```python
from build123d import *

# Parameters (mm, degrees)
F1_DEPTH       = 13
F4_DEPTH       = 3
F5_R           = 1.65
F6_DEPTH       = 1
F8_DEPTH       = 4
F11_DEPTH      = 3
F11_DEPTH_BACK = 2
F12_R          = 1.65
F13_DEPTH      = 3


with BuildPart() as f1:
    # F0 (on Top) → F1 (new body)
    with BuildSketch(Plane.XY):
        with BuildLine():
            Line((0, 0), (5, 0))
            ThreePointArc((5, 0), (10.8477089738, 9.3590674898), (5.4753859206, 18.9988802231))
            Line((5.4753859206, 18.9988802231), (5.4753859206, 43.9988802231))
            Line((5.4753859206, 43.9988802231), (0.649909985, 43.9988802231))
            Line((0.649909985, 43.9988802231), (0.4753859206, 34.0004032716))
            Line((0.4753859206, 34.0004032716), (1.4753859206, 34.0004032716))
            Line((1.4753859206, 34.0004032716), (1.4753859206, 14.2518003603))
            ThreePointArc((1.4753859206, 14.2518003603), (4.7933098793, 8.8839089986), (0, 4.7793922831))
            Line((0, 4.7793922831), (0, 0))
        make_face()
    extrude(amount=F1_DEPTH)

    # F2: F1 across plane


with BuildPart() as f1_1:
    add(f1.part)
    add(f1.part.mirror(Plane.YZ))

    # F3 (on face) → F4 (cut)
    with BuildSketch(Plane.YZ.offset(5.4753859206)):
        Polygon((22.3245644425, 3.6), (25.6731960038, 3.6), (27.3475117844, 6.5), (25.6731960038, 9.4), (22.3245644425, 9.4), (20.6502486618, 6.5), align=None)
    extrude(amount=-F4_DEPTH, mode=Mode.SUBTRACT)

    # F5 (on face) → F6 (cut, through all)
    with BuildSketch(Plane.YZ.offset(2.4753859206)):
        with Locations((23.9988802231, 6.5)):
            Circle(F5_R)
    extrude(amount=-F6_DEPTH, mode=Mode.SUBTRACT)

    # F7 (on face) → F8 (cut, through all)
    with BuildSketch(Plane(origin=(-5.4753859206, 0, 0), x_dir=(0, -1, 0), z_dir=(-1, 0, 0))):
        with BuildLine():
            ThreePointArc((-22.9988802231, 4.85), (-21.3488802231, 6.5), (-22.9988802231, 8.15))
            Line((-22.9988802231, 8.15), (-24.9988802231, 8.15))
            ThreePointArc((-24.9988802231, 8.15), (-26.6488802231, 6.5), (-24.9988802231, 4.85))
            Line((-24.9988802231, 4.85), (-22.9988802231, 4.85))
        make_face()
    extrude(amount=-F8_DEPTH, mode=Mode.SUBTRACT)

    # F10 (on offset) → F11 (cut, two sides)
    with BuildSketch(Plane.XZ.offset(-5)) as f11_sk:
        Polygon((1.7358122868, 3.6363853195), (3.3478692034, 6.5714501963), (1.6120569166, 9.4350648768), (-1.7358122868, 9.3636146805), (-3.3478692034, 6.4285498037), (-1.6120569166, 3.5649351232), align=None)
    extrude(amount=-F11_DEPTH, mode=Mode.SUBTRACT)
    extrude(f11_sk.sketch, amount=F11_DEPTH_BACK, mode=Mode.SUBTRACT)

    # F12 (on face) → F13 (cut, through all)
    with BuildSketch(Plane(origin=(0, 3, 0), x_dir=(-1, 0, 0), z_dir=(0, 1, 0))):
        with Locations((0, 6.5)):
            Circle(F12_R)
    extrude(amount=-F13_DEPTH, mode=Mode.SUBTRACT)

    # F15: sweep along a path in F15_path
    with BuildLine(Plane(origin=(-0.649909985, 43.9988802231, 13), x_dir=(-0.0174524064, 0.9998476952, 0), z_dir=(-0.9998476952, -0.0174524064, 0))) as f15_path:
        Line((0, 0), (-10, 0))
    # F14 (on face) → F15 (sweep, cut)
    with BuildSketch(Plane(origin=(0, 43.9988802231, 0), x_dir=(-1, 0, 0), z_dir=(0, 1, 0))):
        Polygon((0.649909985, 6.5), (1.649909985, 13), (0.449909985, 13), (0.449909985, 0), (1.649909985, 0), align=None)
    sweep(path=f15_path.line, mode=Mode.SUBTRACT)

    # F17: sweep along a path in F17_path
    with BuildLine(Plane(origin=(0.4753859206, 34.0004032716, 13), x_dir=(-0.0174524064, -0.9998476952, 0), z_dir=(0.9998476952, -0.0174524064, 0))) as f17_path:
        Line((0, 0), (-10, 0))
    # F16 (on face) → F17 (sweep)
    with BuildSketch(Plane(origin=(0, 43.9988802231, 0), x_dir=(-1, 0, 0), z_dir=(0, 1, 0))):
        Polygon((-0.649909985, 6.5), (0.350090015, 13), (-1.3149922222, 13), (-1.3149922222, 0), (0.350090015, 0), align=None)
    sweep(path=f17_path.line)


solid = f1_1.part
```
Source: CAD feature listing. Evaluate the final solid. Frame: model axes, mm. A direction names the side the tool comes from. Round coordinates to 2 decimals unless told otherwise and drop trailing zeros. Loops run counter-clockwise (first coordinate to the right, second up) from the corner with the lowest first, then second, coordinate; pieces in that order, holes last. Notation, with made-up numbers: (-7, 68) - (45, 68) arc R14 cw to (45, 75) - close; hole circle Ø3 at (-38.75, -18.75). An arc over 180 degrees is marked (long way). Use CSV: the item, a comma, the result in double quotes.
Q1. Pin query (flat end, axial travel): pin 1 Ø2.5 at (x, z) = (0, 6.5) entering from -Y; pin 2 Ø4.5 at (x, z) = (0.5, 6) entering from +Y; pin 3 Ø6.5 at (y, z) = (26, 9) entering from +X; pin 4 Ø2 at (y, z) = (28, 7.5) entering from -X. Return the tip coordinate at first contact, or that it passes through.
Reported:
pin 1,"y = 34"
pin 2,"y = 44"
pin 3,"x = 5.48"
pin 4,"x = -5.48"
Q2. Ray query, line 1 along X through (y, z) = (30.5, 11.5); line 2 along Z through (x, y) = (0, 2); line 3 along X through (y, z) = (9.5, 9.75). Return the intervals inside material, ascending.
Reported:
line 1,"-5.48 to -1.48, 1.48 to 5.48"
line 2,"0 to 4.85, 8.15 to 13"
line 3,"-10.85 to -4.85, 4.85 to 10.85"
Q3. Section query A-A, the plane x = -4. Output: boundary loops of the cut face in (y, z).
Reported:
outline,"(0, 0) - (6.89, 0) - (6.89, 13) - (0, 13) - close; (12.38, 0) - (44, 0) - (44, 13) - (12.38, 13) - close; hole (23, 4.85) - (25, 4.85) arc R1.65 ccw to (25, 8.15) - (23, 8.15) arc R1.65 ccw to start"
Q4. Section query D-D, the plane y = 40. Output: boundary loops of the cut face in (x, z).
Reported:
outline,"(-5.48, 0) - (-1.58, 0) - (-0.58, 6.5) - (-1.58, 13) - (-5.48, 13) - close; (-0.42, 0) - (5.48, 0) - (5.48, 13) - (-0.42, 13) - (0.58, 6.5) - close"
Q5. Section query B-B, the plane y = 4. Output: boundary loops of the cut face in (x, z).
Reported:
outline,"(-9.28, 0) - (9.28, 0) - (9.28, 13) - (-9.28, 13) - close; hole (-3.35, 6.43) - (-1.61, 3.56) - (1.74, 3.64) - (3.35, 6.57) - (1.61, 9.44) - (-1.74, 9.36) - close"
Q6. Mould query, pull axis Z, two halves, no side actions, for faces 6 (the cylindrical face through (-3.5, 26.65, 6.54)), 7 (the flat face through (3, 22, 0)), 8 (the flat face through (3, 43.999, 6)). Classes: pulls with the +Z half, pulls with the -Z half, needs draft (parallel to the pull), parting line crosses it, or undercut.
Reported:
face 6,"undercut"
face 7,"pulls with the -Z half"
face 8,"needs draft"
Q7. Section query C-C, the plane z = 12.25. Output: boundary loops of the cut face in (x, y).
Reported:
outline,"(-5.48, 19) arc R10.85 ccw to (-5, 0) - (5, 0) arc R10.85 ccw to (5.48, 19) - (5.48, 44) - (-0.23, 44) - (-0.41, 34) - (1.48, 34) - (1.48, 14.25) arc R4.85 cw (long way) to (-1.48, 14.25) - (-1.48, 34) - (-1.36, 34) - (-1.53, 44) - (-5.48, 44) - close"
Q8. Reachability of faces 1 (the flat face through (4, 21.5, 7.97)), 2 (the flat face through (-4, 24, 8.15)), 3 (the cylindrical face through (0.4, 1.5, 4.9)), 4 (the flat face through (1, 34, 6)), 5 (the flat face through (2.53, 4.19, 5.08)) from +Z, -Z, +X, -X, +Y, -Y: full face, straight path, thin tool, end or side. Return the list, or none.
Reported:
face 1,"+X"
face 2,"-X"
face 3,"-Y"
face 4,"+Z, -Z"
face 5,"none"
